Read the model definition and answer for the solid it produces. Units are mm, in the model's axes. A direction names the side the tool comes from. Coordinates: 2 decimals unless noted, no trailing zeros. Loops run counter-clockwise (first coordinate to the right, second up) from the corner with the lowest first, then second, coordinate; pieces in that order, holes last. Notation, with made-up numbers: M 88.25,40 L 120.25,40 A25 ccw 120.25,64 Z; hole C -28.75,1.5 d9. An arc over 180 degrees is marked long. Put each result on its own line as item: value.
Autodesk Inventor part; units mm, degrees
ref_plane "YZ Plane" through (0, 0, 0) normal (1, 0, 0) x (0, 1, 0)
ref_plane "XZ Plane" through (0, 0, 0) normal (0, 1, 0) x (-1, 0, 0)
ref_plane "XY Plane" through (0, 0, 0) normal (0, 0, 1) x (1, 0, 0)
sketch "Sketch1" plane through (0, 0, 0) normal (0, 0, 1) x (1, 0, 0)
  line L0 (0, 0) -> (0, 25.4)
  line L1 (0, 25.4) -> (114.3, 25.4)
  line L2 (114.3, 25.4) -> (114.3, 0)
  line L3 (114.3, 0) -> (0, 0)
  dimension "d0" = 25.4
  dimension "d1" = 114.3
extrude "Extrusion1" add sketch "Sketch1" along normal blind 3.175
sketch "Sketch2" plane through (0, 0, 0) normal (0, 0, -1) x (-1, 0, 0)
  line L0 (-114.3, 0) -> (-114.3, 3.175)
  line L1 (-114.3, 0) -> (-114.3, 25.4)
  line L2 (-114.3, 3.175) -> (0, 3.175)
  line L3 (0, 25.4) -> (0, 0)
  line L4 (0, 3.175) -> (0, 0)
  line L5 (0, 0) -> (-114.3, 0)
  line L6 (0, 0) -> (-114.3, 0)
  line L7 (0, 12.7) -> (-19.05, 12.7)
  line L8 (-114.3, 25.4) -> (-114.3, 22.225)
  line L9 (-114.3, 25.4) -> (-114.3, 0)
  line L10 (0, 0) -> (0, 25.4)
  line L11 (0, 22.225) -> (0, 25.4)
  dimension "d4" = 3.175
extrude "Extrusion2" add sketch "Sketch2" along normal blind 22.225
sketch "Sketch5" plane through (0, 0, 3.175) normal (0, 0, 1) x (1, 0, 0)
  line L0 (0, 0) -> (114.3, 0)
  line L1 (57.15, 0) -> (57.15, 27.3812)
  dimension "d18" = 27.3812
hole "Hole2" at (57.15, 27.3812, 3.175) direction (0, 0, -1) diameter 28.5496 end through all
properties part number "shaft chassis bracket with hole"
1) Straight lines are drawn through the part: line 1 (Y direction, x = 97, z = -20.5) (3 decimals); line 2 (Y direction, x = 46, z = 1.75). For each, find the intervals that lie inside material, in ascending order. Write a range as [from, to].
Answer list:
line 1: y = [0, 3.175]
line 2: y = [0, 18.47]
2) Find section C-C, the plane z = 1.25. Write down the section's boundary in (x, y).
Answer list:
outline: M 0,0 L 114.3,0 L 114.3,25.4 L 71.29,25.4 A14.27 cw 43.01,25.4 L 0,25.4 Z
3) Given pin 1 Ø2 at (x, y) = (83.5, 14.5) entering from -Z; pin 2 Ø6.5 at (x, z) = (80, -13.5) entering from +Y (3 decimals), each flat-ended and moving along its own axis, determine where each tip first touches the part or whether it passes through.
Answer list:
pin 1: stops at z = 0
pin 2: stops at y = 3.175
4) Find section A-A, the plane y = 16.5. Write down the section's boundary in (x, z) (3 decimals).
Answer list:
outline: M 0,0 L 47.91,0 L 47.91,3.175 L 0,3.175 Z; M 66.39,0 L 114.3,0 L 114.3,3.175 L 66.39,3.175 Z
5) Which of the six approach directions +Z, -Z, +X, -X, +Y, -Y give full straight-line access (tool end or side, diameter ignored) to faces 1 (the flat face through (56, 12, 0)), 2 (the flat face through (0, 7, 1))?
Answer list:
face 1: -Z, +X, -X, +Y
face 2: +Z, -Z, -X, +Y, -Y
6) Find section B-B, the plane x = 76. Write down the section's boundary in (y, z) (3 decimals), plus the area to 3 significant figures.
Answer list:
outline: M 0,-22.225 L 3.175,-22.225 L 3.175,0 L 25.4,0 L 25.4,3.175 L 0,3.175 Z
area: 151 mm^2
7) Find section D-D, the plane y = 9. Write down the section's boundary in (x, z) (3 decimals).
Answer list:
outline: M 0,0 L 114.3,0 L 114.3,3.175 L 0,3.175 Z
